Could you check a few things on this model? Use its own coordinates, in mm. A direction names the side the tool comes from. Round coordinates to 2 decimals unless told otherwise and drop trailing zeros. Write each loop counter-clockwise with the first axis right and the second up, starting at its lowest first coordinate (ties: lowest second). Pieces come first, ordered by that corner, then holes. Notation, with made-up numbers: (-26, 65.25) -> (30, 65.25) arc R19 cw to (30, 86.25) -> close; hole circle Ø4 at (68.25, 3.5). An arc over 180 degrees is marked (long way). Answer as CSV lines item,"result". Start each with the question number.
Q1. If I drill on line 1 (Y direction, x = 0, z = -15.85); line 2 (X direction, y = -123.5, z = -9.5); line 3 (Z direction, x = -10, y = -11), over which ranges is the centre line in solid material (lowest first)? Write a range as [from, to].
Q2. Imagine slicing it at B-B on y = -144. Please give me the cut outline in (x, z).
Q3. If we mould it in two halves opening along X, with no side actions, what happens to faces 1 (the cylindrical face through (15.493, -18.346, -1.223)), 2 (the flat face through (15, -79, -3)), 3 (the flat face through (16, -79, -4)), 4 (the flat face through (-16, -79, 4))? For each: pulls with the +X half, pulls with the -X half, needs draft (parallel to the pull), parting line crosses it, or undercut.
Q4. Imagine slicing it at D-D on z = -0.25. Give the number of separate pieces and of enclosed holes in the cut face, and give its area (3 significant figures).
Q5. For faces 5 (the cylindrical face through (-0.33, -82.52, -15.76)), 6 (the flat face through (-15, -79, 3)), which set-ups out of +Z, -Z, +X, -X, +Y, -Y let a thin tool reach every point of the face, with its end or its side?
Q6. Imagine slicing it at A-A on z = -6.5. Please give me the cut outline in (x, y).
Q7. Imagine slicing it at C-C on y = -101.5. Please give me the cut outline in (x, z).
Q8. Will this pin go through, and if not, where does the flat tip stop? pin 1 Ø12 at (x, y) = (-7.5, -21) entering from +Z.
from build123d import *

# Parameters (mm, degrees)
F1_DEPTH = 160
F2_R     = 2.54
F3_DEPTH = 50.8
F4_R     = 2.54
F5_DEPTH = 25.4


with BuildPart() as f1:
    # F0 (on Front) → F1 (new body)
    with BuildSketch(Plane.XZ):
        Polygon((-15, 15.75), (-16, 15.75), (-16, -16.25), (16, -16.25), (16, 15.75), (15, 15.75), (15, -15.25), (-15, -15.25), align=None)
    extrude(amount=F1_DEPTH)

    # F2 (on face) → F3 (cut)
    with BuildSketch(Plane(origin=(-16, 0, 0), x_dir=(0, -1, 0), z_dir=(-1, 0, 0))):
        with Locations((16, -0.25)):
            Circle(F2_R)
        with Locations((48, -0.25)):
            Circle(F2_R)
        with Locations((80, -0.25)):
            Circle(F2_R)
        with Locations((112, -0.25)):
            Circle(F2_R)
        with Locations((144, -0.25)):
            Circle(F2_R)
    extrude(amount=-F3_DEPTH, mode=Mode.SUBTRACT)

    # F4 (on face) → F5 (cut)
    with BuildSketch(Plane(origin=(0, 0, -16.25), x_dir=(1, 0, 0), z_dir=(0, 0, -1))):
        with Locations((0, 144)):
            Circle(F4_R)
        with Locations((0, 112)):
            Circle(F4_R)
        with Locations((0, 80)):
            Circle(F4_R)
        with Locations((0, 48)):
            Circle(F4_R)
        with Locations((0, 16)):
            Circle(F4_R)
    extrude(amount=-F5_DEPTH, mode=Mode.SUBTRACT)


solid = f1.part
Checks:
1,line 1,"[-160, -146.54], [-141.46, -114.54], [-109.46, -82.54], [-77.46, -50.54], [-45.46, -18.54], [-13.46, 0]"
1,line 2,"[-16, -15], [15, 16]"
1,line 3,"[-16.25, -15.25]"
2,outline,"(-16, -16.25) -> (-2.54, -16.25) -> (-2.54, -15.25) -> (-15, -15.25) -> (-15, -2.79) -> (-16, -2.79) -> close; (-16, 2.29) -> (-15, 2.29) -> (-15, 15.75) -> (-16, 15.75) -> close; (2.54, -16.25) -> (16, -16.25) -> (16, -2.79) -> (15, -2.79) -> (15, -15.25) -> (2.54, -15.25) -> close; (15, 2.29) -> (16, 2.29) -> (16, 15.75) -> (15, 15.75) -> close"
3,face 1,"needs draft"
3,face 2,"undercut"
3,face 3,"pulls with the +X half"
3,face 4,"pulls with the -X half"
4,separate pieces,"12"
4,enclosed holes,"0"
4,area,"269 mm^2"
5,face 5,"+Z, -Z"
5,face 6,"+Z, +Y, -Y"
6,outline,"(-16, -160) -> (-15, -160) -> (-15, 0) -> (-16, 0) -> close; (15, -160) -> (16, -160) -> (16, 0) -> (15, 0) -> close"
7,outline,"(-16, -16.25) -> (16, -16.25) -> (16, 15.75) -> (15, 15.75) -> (15, -15.25) -> (-15, -15.25) -> (-15, 15.75) -> (-16, 15.75) -> close"
8,pin 1,"z = -15.25"
